```python
from build123d import *

# Parameters (mm, degrees)
F1_R     = 20
F1_R_2   = 17.55
F4_R     = 17.55
F5_DEPTH = 30
F6_R     = 15
F7_DEPTH = 110.0010001
F8_R     = 20
F8_R_2   = 17
F9_DEPTH = 6
F10_R    = 14


with BuildPart() as f2:
    # F2: sweep along a path in F0
    with BuildLine(Plane.XZ) as f2_path:
        Line((0, 0), (0, -70))
        Line((0, -70), (0, -110))
    # F1 (on Top) → F2 (sweep)
    with BuildSketch(Plane.XY):
        Circle(F1_R)
    sweep(path=f2_path.line)

    # F3: sweep along a path in F0
    with BuildLine(Plane.XZ) as f3_path:
        Line((45, 0), (45, -25))
        Line((45, -25), (0, -70))
    # F1 (on Top) → F3 (sweep)
    with BuildSketch(Plane.XY):
        with Locations((45, 0)):
            Circle(F1_R_2)
    sweep(path=f3_path.line, transition=Transition.RIGHT)

    # F4 (on face) → F5 (cut)
    with BuildSketch(Plane(origin=(0, 0, -110), x_dir=(1, 0, 0), z_dir=(0, 0, -1))):
        Circle(F4_R)
    extrude(amount=-F5_DEPTH, mode=Mode.SUBTRACT)

    # F6 (on face) → F7 (cut, through all)
    with BuildSketch(Plane.XY):
        Circle(F6_R)
    extrude(amount=-F7_DEPTH, mode=Mode.SUBTRACT)

    # F8 (on face) → F9 (cut)
    with BuildSketch(Plane.XY):
        Circle(F8_R)
        Circle(F8_R_2, mode=Mode.SUBTRACT)
    extrude(amount=-F9_DEPTH, mode=Mode.SUBTRACT)

    # F11: sweep along a path in F0
    with BuildLine(Plane.XZ) as f11_path:
        Line((45, 0), (45, -25))
        Line((45, -25), (0, -70))
    # F10 (on face) → F11 (sweep, cut)
    with BuildSketch(Plane.XY):
        with Locations((45, 0)):
            Circle(F10_R)
    sweep(path=f11_path.line, transition=Transition.RIGHT, mode=Mode.SUBTRACT)


solid = f2.part
```
Here's how the part is built. I have some questions about the finished solid (model axes, mm). A direction names the side the tool comes from. Round coordinates to 2 decimals unless told otherwise and drop trailing zeros. Write each loop counter-clockwise with the first axis right and the second up, starting at its lowest first coordinate (ties: lowest second). Pieces come first, ordered by that corner, then holes.
Q1. If we section it at A-A on x = 0: Write out the boundary of the cut face in (y, z).
Q2. Which directions (+Z, -Z, +X, -X, +Y, -Y) give clear straight access to the entire face, cutting with the end or side of a thin tool? Please do faces 1 (the cylindrical face through (35.577, -4.205, -53.308)), 2 (the cylindrical face through (-13.927, 10.679, -95.21)), 3 (the cylindrical face through (61.74, -5.27, -12.78)).
Q3. If we section it at C-C on z = -8: Write out the boundary of the cut face in (x, y).
Q4. If we mould it in two halves opening along X, with no side actions, what happens to faces 4 (the flat face through (0, -18, -110)), 5 (the flat face through (-9, -15, -6))? For each: +X half, -X half, draft (parallel to the pull), parting line (faces both ways), or undercut.
Q5. Will these pins go through, and if not, where does the flat tip stop? P1, Ø2, axis at y = 5.5, z = -41.5, coming from the -X side; P2, Ø22.5, axis at x = 45, y = 0, coming from the -Z side; P3, Ø21, axis at x = 0, y = 0, coming from the -Z side; P4, Ø1, axis at x = 24, y = 9.5, coming from the -Z side.
Q6. Please list where these lines run through material, in increasing order: probe 1 along X at (y, z) = (0, -97); probe 2 along Y at (x, z) = (0, -26.5).
Q7. If we section it at B-B on y = 4.5: Write out the boundary of the cut face in (x, z), plus the area to 3 significant figures.
Answer below:
1. outline: (-20, -110) - (-17.55, -110) - (-17.55, -80) - (-15, -80) - (-15, 0) - (-17, 0) - (-17, -6) - (-20, -6) - close; (15, -80) - (17.55, -80) - (17.55, -110) - (20, -110) - (20, -6) - (17, -6) - (17, 0) - (15, 0) - close
2. face 1: none
2. face 2: -Z
2. face 3: +Z
3. outline: circle Ø40 at (0, 0); circle Ø35.1 at (45, 0); hole circle Ø30 at (0, 0); hole circle Ø28 at (45, 0)
4. face 4: draft
4. face 5: undercut
5. P1: stops at x = -19.49
5. P2: stops at z = -61.07
5. P3: passes through
5. P4: stops at z = -67.54
6. probe 1: x = -20 to -17.55, 17.55 to 20
6. probe 2: y = -20 to -15, 15 to 20
7. outline: (-19.49, -110) - (-16.96, -110) - (-16.96, -80) - (-14.31, -80) - (-14.31, 0) - (-16.39, 0) - (-16.39, -6) - (-19.49, -6) - close; (14.31, -80) - (16.96, -80) - (16.96, -110) - (19.49, -110) - (19.49, -74.5) - (61.96, -32.03) - (61.96, 0) - (58.26, 0) - (58.26, -30.49) - (14.31, -74.44) - close; (14.31, -36.94) - (31.74, -19.51) - (31.74, 0) - (28.04, 0) - (28.04, -17.97) - (19.49, -26.52) - (19.49, -6) - (16.39, -6) - (16.39, 0) - (14.31, 0) - close
7. area: 1,200 mm2
